Input: part model. Units: mm. Frame: model coordinates. Face numbers are marked on the shaded views. A direction names the side the tool comes from. Give positions to 0.01 mm unless a question says otherwise; leave off trailing zeros. Loops run counter-clockwise (first coordinate to the right, second up) from the corner with the lowest first, then second, coordinate; pieces in that order, holes last. Notation, with made-up numbers: M 83,41 L 137,41 A11 ccw 137,56 Z; hole C 74.25,-17.75 d8. An arc over 180 degrees is marked long. Answer as a JSON object with one key per item and string values. Group by question number.
1) First-contact query: P1, Ø6, axis at x = -25, z = 3, coming from the +Y side; P2, Ø8, axis at y = 10, z = 3.5, coming from the +X side; P3, Ø5, axis at y = -4, z = 2.5, coming from the -X side (3 decimals); P4, Ø12, axis at x = -24, y = 11, coming from the -Z side. Flat tips, straight axial feed; report the tip coordinate or a pass-through.
2) Ray query, L1, parallel to Y at x = -18, z = 11.25; L2, parallel to Z at x = -24.5, y = -28; L3, parallel to Y at x = -22, z = 17. Return the intervals inside material, ascending.
3) Section query B-B on y = 0. Return loops of the section in (x, z).
4) Access query for the marked faces 4 and 5. Directions: +Z, -Z, +X, -X, +Y, -Y. A direction counts if a zero-diameter tool reaches every point of the face in a straight line with its end or side. Return the directions, or none.
5) Section query C-C on z = 18.25. Return loops of the section in (x, y), plus the area to 3 significant figures.
6) Section query D-D on z = 1.5. Return loops of the section in (x, y), plus the area to 3 significant figures.
7) Section query A-A on x = 36. Return loops of the section in (y, z), plus the area to 3 significant figures.
8) Draft query along Y for the marked faces 1, 2 and 3. Return one class per face: +Y half, -Y half, draft (parallel to the pull), parting line (faces both ways), or undercut.
from build123d import *

# Parameters (mm, degrees)
SKETCH1_R           = 45
BOSS_EXTRUDE1_DEPTH = 8
SKETCH2_R           = 5
BOSS_EXTRUDE2_DEPTH = 12


with BuildPart() as part:
    # Sketch1 → Boss-Extrude1 (new body)
    with BuildSketch(Plane.XY):
        Circle(SKETCH1_R)
    extrude(amount=BOSS_EXTRUDE1_DEPTH)

    # Sketch2 → Boss-Extrude2 (add)
    with BuildSketch(Plane.XY.offset(8)):
        with Locations((36, 0)):
            Circle(SKETCH2_R)
        with Locations((-18, 31.176914536)):
            Circle(SKETCH2_R)
        with Locations((-18, -31.176914536)):
            Circle(SKETCH2_R)
    extrude(amount=BOSS_EXTRUDE2_DEPTH)


solid = part.part
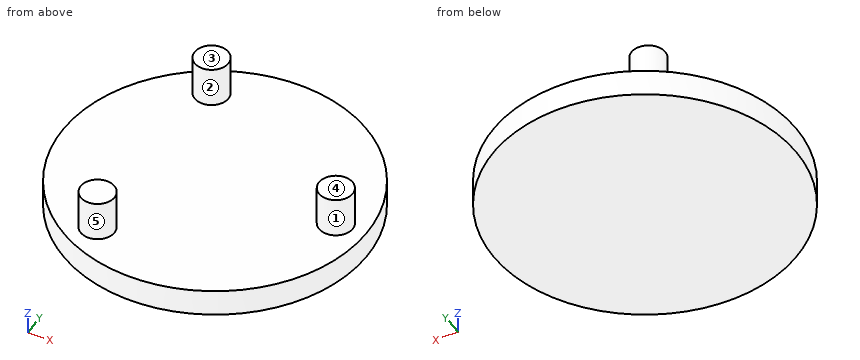
Output:
{
 "1": {"P1": "stops at y = 39.26", "P2": "stops at x = 44.6", "P3": "stops at x = -44.975", "P4": "stops at z = 0"},
 "2": {"L1": "y = -36.18 to -26.18, 26.18 to 36.18", "L2": "z = 0 to 8", "L3": "y = -34.18 to -28.18, 28.18 to 34.18"},
 "3": {"outline": "M -45,0 L 45,0 L 45,8 L 41,8 L 41,20 L 31,20 L 31,8 L -45,8 Z"},
 "4": {"face 4": "+Z, +X, -X, +Y, -Y", "face 5": "+Z"},
 "5": {"outline": "C -18,-31.18 d10; C -18,31.18 d10; C 36,0 d10", "area": "236 mm^2"},
 "6": {"outline": "C 0,0 d90", "area": "6,360 mm^2"},
 "7": {"outline": "M -27,0 L 27,0 L 27,8 L 5,8 L 5,20 L -5,20 L -5,8 L -27,8 Z", "area": "552 mm^2"},
 "8": {"face 1": "parting line", "face 2": "undercut", "face 3": "draft"}
}
